```python
from build123d import *

# Parameters (mm, degrees)
F2_DEPTH = 63.5
F3_DEPTH = 25.4


with BuildPart() as f2:
    # F0 (on Front) → F2 (new body, symmetric)
    with BuildSketch(Plane.XZ):
        Polygon((-41.275, -9.525), (41.275, -9.525), (41.275, 9.525), (22.225, 9.525), (-41.275, 9.525), align=None)
    extrude(amount=F2_DEPTH, both=True)

    # F1 (on face) → F3 (join, symmetric)
    with BuildSketch(Plane.XZ):
        with BuildLine():
            Line((22.225, 27.0002), (22.225, 9.525))
            Line((22.225, 9.525), (41.275, 9.525))
            Line((41.275, 9.525), (41.275, 27.0002))
            ThreePointArc((41.275, 27.0002), (45.92468, 38.22552), (57.15, 42.8752))
            Line((57.15, 42.8752), (70.925324, 42.8752))
            Line((70.925324, 42.8752), (70.925324, 61.9252))
            Line((70.925324, 61.9252), (57.15, 61.9252))
            ThreePointArc((57.15, 61.9252), (32.454296, 51.695904), (22.225, 27.0002))
        make_face()
    extrude(amount=F3_DEPTH, both=True)


solid = f2.part
```
Geometry check sheet. Reference: the model listing, model coordinates, mm. A direction names the side the tool comes from. Coordinates: 2 decimals unless noted, no trailing zeros. Write each loop counter-clockwise with the first axis right and the second up, starting at its lowest first coordinate (ties: lowest second). Pieces come first, ordered by that corner, then holes. Notation, with made-up numbers: M -5,39.25 L 31,39.25 A25 cw 31,70.25 Z; hole C -14,31.5 d6. An arc over 180 degrees is marked long. One line per item, written item: value. Start each with the question number.
(1) Sectioned sample at A-A, the plane y = 19.5. Enter the section's corners in (x, z) (3 decimals), and give its area (3 significant figures).
(2) Scan lines: line 1 along Z through (x, y) = (14, -55) (3 decimals); line 2 along X through (y, z) = (27, 0.5) (3 decimals); line 3 along X through (y, z) = (14, 17) (3 decimals). Record each from-to range of solid material in increasing order. Write a range as [from, to].
(3) Sectioned sample at C-C, the plane z = -3. Enter the section's corners in (x, y) (3 decimals).
(4) Tool access check on faces 1 (the face through (41, -25.4, 36)), 2 (the face through (41, 25.4, 36)), 3 (the face through (41.275, -1, 4)). Record the directions out of +Z, -Z, +X, -X, +Y, -Y that give a thin tool (end or side, any length) a straight path to the whole face; none if there is none.
(5) Sectioned sample at B-B, the plane x = 60. Enter the section's corners in (y, z).
(6) Depth check by flat-ended pin: pin 1 (11 mm diameter, centred on x = 66.5, y = -8, fed in from -Z); pin 2 (3 mm diameter, centred on y = 7.5, z = 10, fed in from -X) (3 decimals); pin 3 (14 mm diameter, centred on y = 9.5, z = 18, fed in from -X) (3 decimals); pin 4 (1.5 mm diameter, centred on x = -26, y = -10, fed in from +Z) (3 decimals). Enter the tip coordinate at first touch or a pass-through.
Filled sheet:
1. outline: M -41.275,-9.525 L 41.275,-9.525 L 41.275,27 A15.875 cw 57.15,42.875 L 70.925,42.875 L 70.925,61.925 L 57.15,61.925 A34.925 ccw 22.225,27 L 22.225,9.525 L -41.275,9.525 Z
1. area: 2,930 mm²
2. line 1: [-9.525, 9.525]
2. line 2: [-41.275, 41.275]
2. line 3: [22.225, 41.275]
3. outline: M -41.275,-63.5 L 41.275,-63.5 L 41.275,63.5 L -41.275,63.5 Z
4. face 1: +Z, +X, -X, -Y
4. face 2: +Z, +X, -X, +Y
4. face 3: -Z, +X, +Y, -Y
5. outline: M -25.4,42.88 L 25.4,42.88 L 25.4,61.93 L -25.4,61.93 Z
6. pin 1: z = 42.88
6. pin 2: x = -41.275
6. pin 3: x = 22.225
6. pin 4: z = 9.525
